```python
from build123d import *

# Parameters (mm, degrees)
F1_DEPTH = 30
F2_R     = 2


with BuildPart() as f1:
    # F0 (on Front) → F1 (new body)
    with BuildSketch(Plane.XZ):
        Polygon((-23, 0), (0, 0), (24, 0), (24, 10.1), (19, 10.1), (19, 8.1), (21, 8.1), (21, 3), (0, 3), (-20, 3), (-20, 8.1), (-14.3, 8.1), (-14.3, 10.1), (-23, 10.1), align=None)
    extrude(amount=F1_DEPTH)

    # F2
    f2_edges = [f1.edges().sort_by_distance(p)[0] for p in [
        (-23, -15, 10.1),
        (24, -15, 10.1),
        (-23, -15, 0),
        (24, -15, 0),
    ]]
    fillet(f2_edges, radius=F2_R)


solid = f1.part
```
Geometry check sheet. Reference: the model listing, model coordinates, mm. A direction names the side the tool comes from. Coordinates: 2 decimals unless noted, no trailing zeros. Order: outer loops, then holes, each group sorted by start corner. A loop starts at its lowest first (then second) coordinate and runs counter-clockwise, first axis right, second up. Notation, with made-up numbers: (32.5, -16) - (70.5, -16) arc R26 ccw to (70.5, 0) - close; hole circle Ø4 at (88.25, 17.25). An arc over 180 degrees is marked (long way). Answer in a Markdown table with one row per item. Add a question column.
1. Section check B-B (z = 5.5). Enter the section's corners in (x, y), plus the area to 3 significant figures.
2. Section check A-A (x = -17.5). Enter the section's corners in (y, z), plus the area to 3 significant figures.
3. Material ranges on L1, parallel to Z at x = 20, y = -14; L2, parallel to X at y = -11.25, z = 7.5; L3, parallel to Z at x = -12, y = -12.5, recorded low to high. Write a range as [from, to].
4. Gauge pin test, flat ends, axial feed: pin 1 Ø1 at (y, z) = (-16, 9) entering from -X; pin 2 Ø3 at (x, y) = (9, -7) entering from +Z; pin 3 Ø1.6 at (y, z) = (-17, 9) entering from +X. Record the tip position at first contact, or that the pin passes through.
5. Section check D-D (x = -3.5). Enter the section's corners in (y, z).
6. Section check C-C (y = -23). Enter the section's corners in (x, z).
7. Draft check along Z on faces 4 (the face through (19, -15, 9)), 5 (the face through (-22.4, -15.21, 0.57)), 6 (the face through (-17, -15, 8.1)). Enter one of: +Z half, -Z half, draft (parallel to the pull), parting line (faces both ways), or undercut.
8. Access from +Z, -Z, +X, -X, +Y, -Y to the whole of each face (thin tool, end or side, straight path). Record for faces 1 (the face through (-22.4, -15.21, 9.53)), 2 (the face through (-14.3, -15, 9)), 3 (the face through (21, -15, 6)).
Data:
| question | item | result |
|---|---|---|
| 1 | outline | (-23, -30) - (-20, -30) - (-20, 0) - (-23, 0) - close; (21, -30) - (24, -30) - (24, 0) - (21, 0) - close |
| 1 | area | 180 mm² |
| 2 | outline | (-30, 0) - (0, 0) - (0, 3) - (-30, 3) - close; (-30, 8.1) - (0, 8.1) - (0, 10.1) - (-30, 10.1) - close |
| 2 | area | 150 mm² |
| 3 | L1 | z = [0, 3], [8.1, 10.1] |
| 3 | L2 | x = [-23, -20], [21, 24] |
| 3 | L3 | z = [0, 3] |
| 4 | pin 1 | stops at x = -22.96 |
| 4 | pin 2 | stops at z = 3 |
| 4 | pin 3 | stops at x = 24 |
| 5 | outline | (-30, 0) - (0, 0) - (0, 3) - (-30, 3) - close |
| 6 | outline | (-23, 2) arc R2 ccw to (-21, 0) - (22, 0) arc R2 ccw to (24, 2) - (24, 8.1) arc R2 ccw to (22, 10.1) - (19, 10.1) - (19, 8.1) - (21, 8.1) - (21, 3) - (-20, 3) - (-20, 8.1) - (-14.3, 8.1) - (-14.3, 10.1) - (-21, 10.1) arc R2 ccw to (-23, 8.1) - close |
| 7 | face 4 | draft |
| 7 | face 5 | -Z half |
| 7 | face 6 | undercut |
| 8 | face 1 | +Z, -X, +Y, -Y |
| 8 | face 2 | +Z, +Y, -Y |
| 8 | face 3 | +Y, -Y |
